from build123d import *

# Parameters (mm, degrees)
BOSS_EXTRUDE1_DEPTH        = 3.125
CUT_EXTRUDE1_DEPTH         = 195.919695848
F_6_0_6_DIAMETER_HOLE1_D   = 6
F_2_5_2_5_DIAMETER_HOLE1_D = 2.5
F_4_2_4_2_DIAMETER_HOLE1_D = 4.2


with BuildPart() as part:
    # Sketch1 → Boss-Extrude1 (new body)
    with BuildSketch(Plane.XZ.offset(-108.650350882)):
        with BuildLine():
            Line((43.23749287, 110.033281417), (43.23749287, 185.037999923))
            ThreePointArc((43.23749287, 185.037999923), (41.773026776, 188.573533829), (38.23749287, 190.037999923))
            Line((38.23749287, 190.037999923), (7.999992871, 190.037999923))
            ThreePointArc((7.999992871, 190.037999923), (2.343138621, 187.694854172), (-7.129e-06, 182.037999923))
            Line((-7.129e-06, 182.037999923), (-7.129e-06, 178.037999923))
            ThreePointArc((-7.129e-06, 178.037999923), (2.343138621, 172.381145673), (7.999992871, 170.037999923))
            Line((7.999992871, 170.037999923), (15.604000266, 170.037999923))
            Line((15.604000266, 170.037999923), (15.604000266, 162.405058673))
            ThreePointArc((15.604000266, 162.405058673), (15.379885206, 161.485149612), (14.757767585, 160.771406025))
            ThreePointArc((14.757767585, 160.771406025), (13.383453483, 159.667684666), (12.155505046, 158.40313624))
            ThreePointArc((12.155505046, 158.40313624), (11.856365467, 156.265617566), (13.673543586, 155.100999923))
            Line((13.673543586, 155.100999923), (16.979195581, 155.100999923))
            ThreePointArc((16.979195581, 155.100999923), (31.499992871, 149.100999923), (16.979195581, 143.100999923))
            Line((16.979195581, 143.100999923), (13.673543586, 143.100999923))
            ThreePointArc((13.673543586, 143.100999923), (11.856365467, 141.93638228), (12.155505046, 139.798863605))
            ThreePointArc((12.155505046, 139.798863605), (12.809817923, 139.086361098), (13.510844612, 138.419767711))
            ThreePointArc((13.510844612, 138.419767711), (15.615996699, 133.891251825), (19.774392147, 131.125954603))
            ThreePointArc((19.774392147, 131.125954603), (22.280047532, 129.310425898), (23.23749287, 126.368020113))
            Line((23.23749287, 126.368020113), (23.23749287, 110.033281417))
            ThreePointArc((23.23749287, 110.033281417), (33.23749287, 100.033281417), (43.23749287, 110.033281417))
        make_face()
    extrude(amount=-BOSS_EXTRUDE1_DEPTH)

    # Sketch2 → Cut-Extrude1 (cut, through all)
    with BuildSketch(Plane(origin=(0, 111.775350882, 0), x_dir=(-1, 0, 0), z_dir=(0, 1, 0))):
        with BuildLine():
            Line((-43.23749287, 123.037999923), (-43.23749287, 117.037999923))
            Line((-43.23749287, 117.037999923), (-33.23749287, 117.037999923))
            ThreePointArc((-33.23749287, 117.037999923), (-30.23749287, 120.037999923), (-33.23749287, 123.037999923))
            Line((-33.23749287, 123.037999923), (-43.23749287, 123.037999923))
        make_face()
    extrude(amount=-CUT_EXTRUDE1_DEPTH, mode=Mode.SUBTRACT)

    # Ø6.0 (6) Diameter Hole1 (through all)
    with Locations(Plane(origin=(0, 108.650350882, 0), x_dir=(-1, 0, 0), z_dir=(0, -1, 0))):
        with Locations((-10.73749287, -180.037999923), (-35.73749287, -180.037999923)):
            Hole(F_6_0_6_DIAMETER_HOLE1_D / 2)

    # Ø2.5 (2.5) Diameter Hole1 (through all)
    with Locations(Plane(origin=(0, 108.650350882, 0), x_dir=(-1, 0, 0), z_dir=(0, -1, 0))):
        with Locations((-34.048992871, -149.100999923), (-17.475492871, -158.669714609), (-17.475492871, -139.532285236)):
            Hole(F_2_5_2_5_DIAMETER_HOLE1_D / 2)

    # Ø4.2 (4.2) Diameter Hole1 (through all)
    with Locations(Plane(origin=(0, 108.650350882, 0), x_dir=(-1, 0, 0), z_dir=(0, -1, 0))):
        with Locations((-33.23749287, -104.211683364)):
            Hole(F_4_2_4_2_DIAMETER_HOLE1_D / 2)


solid = part.part
Can you work these out from the model? Positions are in its coordinate system, mm. A direction names the side the tool comes from. Coordinates: 2 decimals unless noted, no trailing zeros. Loops run counter-clockwise (first coordinate to the right, second up) from the corner with the lowest first, then second, coordinate; pieces in that order, holes last. Notation, with made-up numbers: (47, 11) - (71, 11) arc R24 cw to (71, 37) - close; hole circle Ø1 at (-36.5, 74). An arc over 180 degrees is marked (long way). Answer as a JSON object with one key per item and string values. Group by question number.
Item 1: If we section it at B-B (y = 110.8): State how many separate pieces and enclosed holes the cut face has, plus the area to 3 significant figures.
Item 2: On a 3-axis mill with a long thin cutter (end or side, diameter ignored), from which of +Z, -Z, +X, -X, +Y, -Y can I reach the whole of each face in a straight line? I mean faces 1 (the face through (15.386, 110.191, 161.497)), 2 (the face through (43.237, 110, 154)), 3 (the face through (38, 110, 117.038)). Say none if no direction works.
Item 3: If we section it at C-C (x = 28.5): List the corners of the cut face in (y, z) for me.
Item 4: If I drill on L1, parallel to Z at x = 36.5, y = 109.9; L2, parallel to Z at x = 10.5, y = 110.55; L3, parallel to Z at x = 33, y = 109, over which ranges is the centre line in solid material (lowest first)? Write a range as from..to.
Item 5: If we section it at A-A (x = 22): List the corners of the cut face in (y, z) for me.
Item 6: For pin 1 (5.5 mm diameter, centred on x = 33.24, z = 104.21, fed in from +Y); pin 2 (1.6 mm diameter, centred on y = 111, z = 167.5, fed in from -X); pin 3 (0.9 mm diameter, centred on x = 37, y = 110, fed in from -Z); pin 4 (1.5 mm diameter, centred on y = 110, z = 124.5, fed in from -X), each with a flat end and sliding along its axis, tell me the tip position at first contact or that it passes through.
Item 7: If we section it at D-D (z = 167): List the corners of the cut face in (x, y) for me, plus the area to 3 significant figures.
Item 8: If we mould it in two halves opening along X, with no side actions, what happens to faces 4 (the face through (38, 110, 123.038)), 5 (the face through (15.604, 110, 166)), 6 (the face through (33.78, 110.23, 150.32))? For each: released by +X, released by -X, zero draft, split by the parting line, or undercut.
Returned:
{
 "1": {"separate pieces": "1", "enclosed holes": "6", "area": "2,140 mm²"},
 "2": {"face 1": "-X, +Y, -Y", "face 2": "+Z, -Z, +X, +Y, -Y", "face 3": "+X, +Y, -Y"},
 "3": {"outline": "(108.65, 101.23) - (111.78, 101.23) - (111.78, 142.62) - (108.65, 142.62) - close; (108.65, 155.58) - (111.78, 155.58) - (111.78, 190.04) - (108.65, 190.04) - close"},
 "4": {"L1": "z = 100.58..117.04, 123.04..177.14, 182.94..190.04", "L2": "z = 170.04..177.05, 183.03..190.04", "L3": "z = 100.04..102.13, 106.3..117.05, 123.03..148.42, 149.78..178.81, 181.27..190.04"},
 "5": {"outline": "(108.65, 129.66) - (111.78, 129.66) - (111.78, 140.66) - (108.65, 140.66) - close; (108.65, 157.54) - (111.78, 157.54) - (111.78, 190.04) - (108.65, 190.04) - close"},
 "6": {"pin 1": "stops at y = 111.78", "pin 2": "stops at x = 15.6", "pin 3": "stops at z = 100.6", "pin 4": "stops at x = 23.24"},
 "7": {"outline": "(15.6, 108.65) - (43.24, 108.65) - (43.24, 111.78) - (15.6, 111.78) - close", "area": "86.4 mm²"},
 "8": {"face 4": "zero draft", "face 5": "released by -X", "face 6": "undercut"}
}
